Check sheet for the modelled part. Datum: model origin and axes. Units: mm. Face numbers are marked on the shaded views. Round coordinates to 2 decimals unless told otherwise and drop trailing zeros. Loops run counter-clockwise (first coordinate to the right, second up) from the corner with the lowest first, then second, coordinate; pieces in that order, holes last. Notation, with made-up numbers: (32, 17) -> (67, 17) arc R25 cw to (67, 44) -> close; hole circle Ø5 at (61, 50). An arc over 180 degrees is marked (long way). One line per question, with ' | ' between items.
```python
from build123d import *

# Parameters (mm, degrees)
SKETCH1_W           = 220
SKETCH1_H           = 220
BOSS_EXTRUDE1_DEPTH = 5
BOSS_EXTRUDE2_DEPTH = 21
BOSS_EXTRUDE3_DEPTH = 5


with BuildPart() as part:
    # Sketch1 → Boss-Extrude1 (new body)
    with BuildSketch(Plane(origin=(0, 0, 0), x_dir=(1, 0, 0), z_dir=(0, 1, 0))):
        Rectangle(SKETCH1_W, SKETCH1_H)
    extrude(amount=BOSS_EXTRUDE1_DEPTH)

    # Sketch2 → Boss-Extrude2 (add)
    with BuildSketch(Plane(origin=(0, 5, 0), x_dir=(1, 0, 0), z_dir=(0, 1, 0))):
        Polygon((-40, 110), (40, 110), (40, 100), (-30, 100), (-30, 53), (110, 53), (110, 43), (-40, 43), align=None)
    extrude(amount=BOSS_EXTRUDE2_DEPTH)

    # Sketch3 → Boss-Extrude3 (add)
    with BuildSketch(Plane(origin=(0, 5, 0), x_dir=(1, 0, 0), z_dir=(0, 1, 0))):
        Polygon((-110, 38), (110, 38), (110, 26.532503788), (-95, 26.532503788), (-95, -78.467496212), (110, -78.467496212), (110, -90.467496212), (-110, -90.467496212), align=None)
    extrude(amount=BOSS_EXTRUDE3_DEPTH)


solid = part.part
```
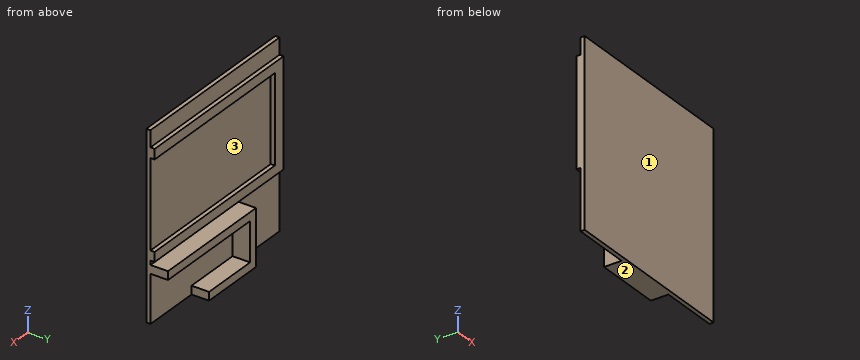
(1) Sectioned sample at C-C, the plane z = 6. Record the cut outline in (x, y).
Answer:
outline: (-110, 0) -> (110, 0) -> (110, 5) -> (-95, 5) -> (-95, 10) -> (-110, 10) -> close
(2) Sectioned sample at A-A, the plane y = 17. Record the cut outline in (x, z).
Answer:
outline: (-40, -110) -> (40, -110) -> (40, -100) -> (-30, -100) -> (-30, -53) -> (110, -53) -> (110, -43) -> (-40, -43) -> close
(3) Sectioned sample at B-B, the plane x = -56. Record the cut outline in (y, z).
Answer:
outline: (0, -110) -> (5, -110) -> (5, -38) -> (10, -38) -> (10, -26.53) -> (5, -26.53) -> (5, 78.47) -> (10, 78.47) -> (10, 90.47) -> (5, 90.47) -> (5, 110) -> (0, 110) -> close
(4) Sectioned sample at D-D, the plane x = 95. Record the cut outline in (y, z), and give its area (3 significant figures).
Answer:
outline: (0, -110) -> (5, -110) -> (5, -53) -> (26, -53) -> (26, -43) -> (5, -43) -> (5, -38) -> (10, -38) -> (10, -26.53) -> (5, -26.53) -> (5, 78.47) -> (10, 78.47) -> (10, 90.47) -> (5, 90.47) -> (5, 110) -> (0, 110) -> close | area: 1,430 mm2
(5) Go/stop test with flat-tipped pins: pin 1 (6.5 mm diameter, centred on y = 17.5, z = -66.5, fed in from +X); pin 2 (21.5 mm diameter, centred on x = 30.5, z = -70, fed in from +Y); pin 3 (21.5 mm diameter, centred on x = -17.5, z = 99, fed in from +Y). Record where each tip stops, or that it passes through.
Answer:
pin 1: stops at x = -30 | pin 2: stops at y = 5 | pin 3: stops at y = 10
(6) Scan lines: probe 1 along Z at (x, y) = (10.5, 5.5); probe 2 along Z at (x, y) = (-6, 20); probe 3 along Z at (x, y) = (-86, 5.5). Record each from-to range of solid material in increasing order.
Answer:
probe 1: z = -110 to -100, -53 to -43, -38 to -26.53, 78.47 to 90.47 | probe 2: z = -110 to -100, -53 to -43 | probe 3: z = -38 to -26.53, 78.47 to 90.47
(7) Mould release check, pull along Z, two halves, no side actions. Record for the marked faces 1, 2 and 3: +Z half, -Z half, draft (parallel to the pull), parting line (faces both ways), or undercut.
Answer:
face 1: draft | face 2: -Z half | face 3: undercut
